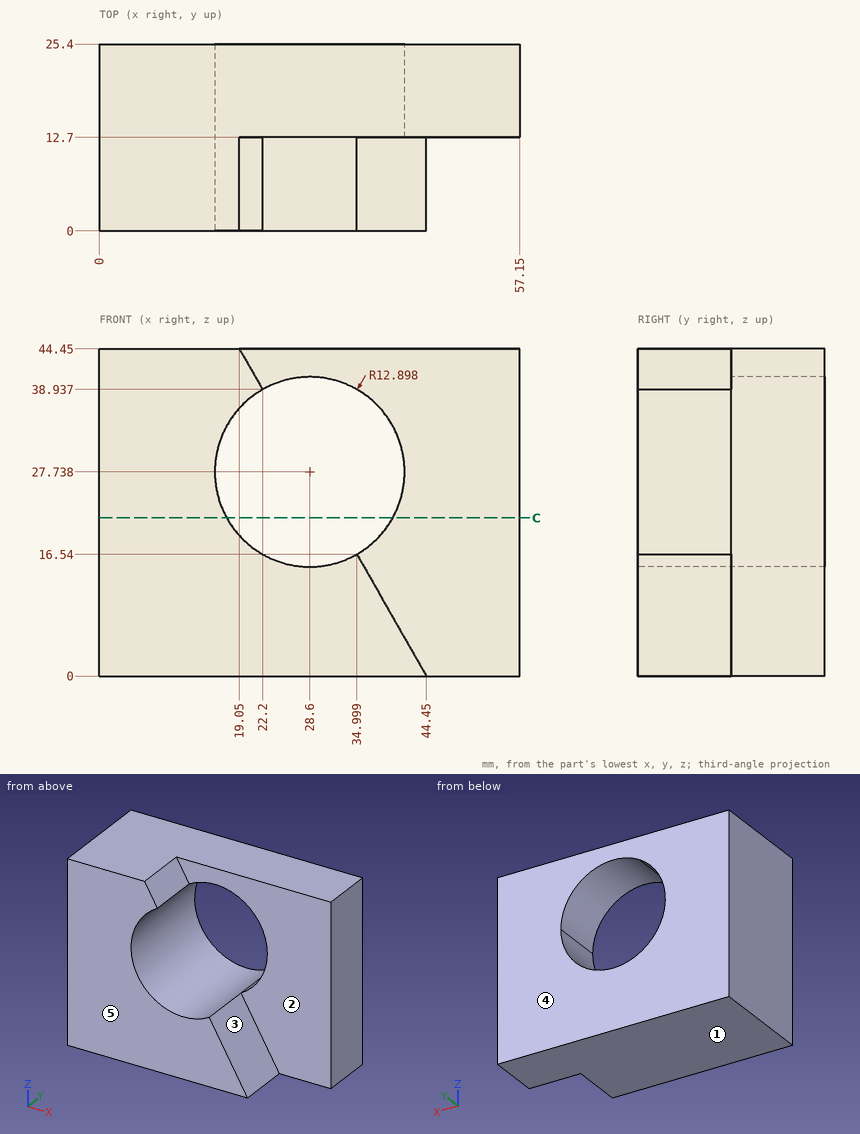
Input: dimensioned drawing with shaded views. Units: mm. Origin: part minimum x, y, z. A direction names the side the tool comes from. Coordinates: 2 decimals unless noted, no trailing zeros. Loops run counter-clockwise (first coordinate to the right, second up) from the corner with the lowest first, then second, coordinate; pieces in that order, holes last. Notation, with made-up numbers: M 84.5,-29 L 122.5,-29 A20 ccw 122.5,7 Z; hole C 23,-3 d11. An arc over 180 degrees is marked long. Use a Markdown table: item, result. Add a question column.
1) Pin query (flat end, axial travel): P1, Ø1, axis at y = 3.5, z = 12.5, coming from the -X side; P2, Ø1, axis at x = 40, z = 9.5, coming from the -Y side. Return the tip coordinate at first contact, or that it passes through.
2) Section C-C, the plane z = 21.5. Return the cut outline in (x, y).
3) Set-up query: the marked faces 1 and 2. Return all of +Z, -Z, +X, -X, +Y, -Y with unobstructed straight access to the full face (end or side cutting, diameter ignored); none if empty.
4) Line query: L1, parallel to X at y = 15.75, z = 18.5; L2, parallel to Y at x = 29.5, z = 42; L3, parallel to X at y = 13, z = 26. Output: solid intervals per line, ascending. Write a range as from..to.
5) Draft query along Y for the marked faces 3, 4 and 5. Return one class per face: +Y half, -Y half, draft (parallel to the pull), parting line (faces both ways), or undercut.
Answer below:
| question | item | result |
|---|---|---|
| 1 | P1 | x = 0 |
| 1 | P2 | y = 12.7 |
| 2 | outline | M 0,0 L 17.31,0 L 17.31,25.4 L 0,25.4 Z; M 39.89,12.7 L 57.15,12.7 L 57.15,25.4 L 39.89,25.4 Z |
| 3 | face 1 | -Z, +X, -X, +Y, -Y |
| 3 | face 2 | +Z, +X, -Y |
| 4 | L1 | 0..19.6, 37.6..57.15 |
| 4 | L2 | 12.7..25.4 |
| 4 | L3 | 0..15.82, 41.38..57.15 |
| 5 | face 3 | draft |
| 5 | face 4 | +Y half |
| 5 | face 5 | -Y half |
